Could you check a few things on this model? Use its own coordinates, in mm. A direction names the side the tool comes from. Coordinates: 2 decimals unless noted, no trailing zeros. Loops run counter-clockwise (first coordinate to the right, second up) from the corner with the lowest first, then second, coordinate; pieces in that order, holes last.
1) Imagine slicing it at A-A on z = 19. Please give me the cut outline in (x, y) (3 decimals).
2) Will these pins go through, and if not, where does the flat tip stop? P1, Ø5, axis at y = 7.5, z = 20.5, coming from the +X side; P2, Ø12, axis at x = 3.5, y = -8.5, coming from the +Z side; P3, Ø8, axis at x = 6, z = 14, coming from the -Y side; P4, Ø11, axis at y = 0, z = 19, coming from the -X side.
3) Imagine slicing it at D-D on z = 3. Please give me the cut outline in (x, y), plus the area to 3 significant figures.
4) For faces 5 (the face through (-1.13, 1.84, 10.7)), 6 (the face through (12.01, -16.07, 1.97)), 7 (the face through (3, -2, 14)), which set-ups out of +Z, -Z, +X, -X, +Y, -Y let a thin tool reach every point of the face, with its end or its side?
5) Imagine slicing it at C-C on x = 12.75. Please give me the cut outline in (y, z), plus the area to 3 significant figures.
6) If I drill on line 1 along Z through (x, y) = (2, 0) (3 decimals); line 2 along Z through (x, y) = (-6.5, -10); line 3 along X through (y, z) = (-8.5, 15.25), over which ranges is the centre line in solid material (lowest first)?
7) Thinking about a two-plate mould opening in Y: for faces 1 (the face through (-13.49, 9.43, 1.97)), 2 (the face through (17, -17.07, 2.03)), 3 (the face through (17.63, 18.15, 2.76)), 4 (the face through (-3, 5, 11)), which applies, released by +Y, released by -Y, zero draft, split by the parting line, or undercut?
8) Imagine slicing it at B-B on y = 12.75. Please give me the cut outline in (x, z), plus the area to 3 significant figures.
```python
from build123d import *

# Parameters (mm, degrees)
F0_W     = 37
F0_H     = 37
F0_R     = 3.4
F1_DEPTH = 4
F3_DEPTH = 25
F5_DEPTH = 37.001
F7_DEPTH = 21.501
F8_R     = 8.5
F9_DEPTH = 3.8
F10_R    = 5
F11_R    = 2


with BuildPart() as f1:
    # F0 (on Top) → F1 (new body)
    with BuildSketch(Plane.XY):
        Rectangle(F0_W, F0_H)
        with Locations((12.75, -12.75)):
            Circle(F0_R, mode=Mode.SUBTRACT)
        with Locations((-12.75, 12.75)):
            Circle(F0_R, mode=Mode.SUBTRACT)
    extrude(amount=F1_DEPTH)

    # F2 (on face) → F3 (join)
    with BuildSketch(Plane.XY.offset(4)):
        Polygon((-18.5, -13.5), (-18.5, -18.5), (3, -18.5), (3, 13.5), (18.5, 13.5), (18.5, 18.5), (-3, 18.5), (-3, -13.5), align=None)
    extrude(amount=F3_DEPTH)

    # F4 (on face) → F5 (cut, through all)
    with BuildSketch(Plane.XZ.offset(18.5)):
        Polygon((-3, 29), (-18.5, 29), (-18.5, 4), align=None)
        Polygon((18.5, 29), (3, 29), (18.5, 4), align=None)
    extrude(amount=-F5_DEPTH, mode=Mode.SUBTRACT)

    # F6 (on face) → F7 (cut, through all)
    with BuildSketch(Plane(origin=(-3, 0, 0), x_dir=(0, -1, 0), z_dir=(-1, 0, 0))):
        with BuildLine():
            Line((3.1448370387, 22.725), (-3.1448370387, 22.725))
            ThreePointArc((-3.1448370387, 22.725), (0, 14.125), (3.1448370387, 22.725))
        make_face()
    extrude(amount=-F7_DEPTH, mode=Mode.SUBTRACT)

    # F8 (on face) → F9 (cut)
    with BuildSketch(Plane(origin=(-3, 0, 0), x_dir=(0, -1, 0), z_dir=(-1, 0, 0))):
        with Locations((0, 19)):
            Circle(F8_R)
    extrude(amount=-F9_DEPTH, mode=Mode.SUBTRACT)

    # F10
    f10_edges = [f1.edges().sort_by_distance(p)[0] for p in [
        (-18.5, 18.5, 2),
        (18.5, -18.5, 2),
    ]]
    fillet(f10_edges, radius=F10_R)

    # F11
    f11_edges = [f1.edges().sort_by_distance(p)[0] for p in [
        (0, -18.5, 29),
        (0, 18.5, 29),
        (-18.5, -18.5, 2),
        (18.5, 18.5, 2),
        (-3, 18.5, 16.5),
        (3, -18.5, 16.5),
    ]]
    fillet(f11_edges, radius=F11_R)


solid = f1.part
```
Filled in:
1. outline: (-9.2, -18.5) - (1, -18.5) arc R2 ccw to (3, -16.5) - (3, -4.875) - (0.8, -4.875) - (0.8, -8.5) - (-3, -8.5) - (-3, -13.5) - (-9.2, -13.5) - close; (-3, 8.5) - (0.8, 8.5) - (0.8, 4.875) - (3, 4.875) - (3, 13.5) - (9.2, 13.5) - (9.2, 18.5) - (-1, 18.5) arc R2 ccw to (-3, 16.5) - close
2. P1: stops at x = 3
2. P2: stops at z = 29
2. P3: stops at y = -18.23
2. P4: stops at x = 0.8
3. outline: (-18.5, -16.5) arc R2 ccw to (-16.5, -18.5) - (13.5, -18.5) arc R5 ccw to (18.5, -13.5) - (18.5, 16.5) arc R2 ccw to (16.5, 18.5) - (-13.5, 18.5) arc R5 ccw to (-18.5, 13.5) - close; hole circle Ø6.8 at (-12.75, 12.75); hole circle Ø6.8 at (12.75, -12.75)
3. area: 1,280 mm2
4. face 5: -X
4. face 6: +Z, -Z
4. face 7: +Z, +X, -Y
5. outline: (-18.5, 0) - (-16.15, 0) - (-16.15, 4) - (-18.5, 4) - close; (-9.35, 0) - (18.5, 0) - (18.5, 13.27) - (13.5, 13.27) - (13.5, 4) - (-9.35, 4) - close
5. area: 167 mm2
6. line 1: z = 0 to 14.125, 22.725 to 29
6. line 2: z = 0 to 4
6. line 3: x = -3 to 3
7. face 1: undercut
7. face 2: released by -Y
7. face 3: released by +Y
7. face 4: zero draft
8. outline: (-18.5, 0) - (-16.15, 0) - (-16.15, 4) - (-18.5, 4) - close; (-9.35, 0) - (18.5, 0) - (18.5, 4) - (3, 4) - (3, 29) - (-3, 29) - (-3, 4) - (-9.35, 4) - close
8. area: 271 mm2
